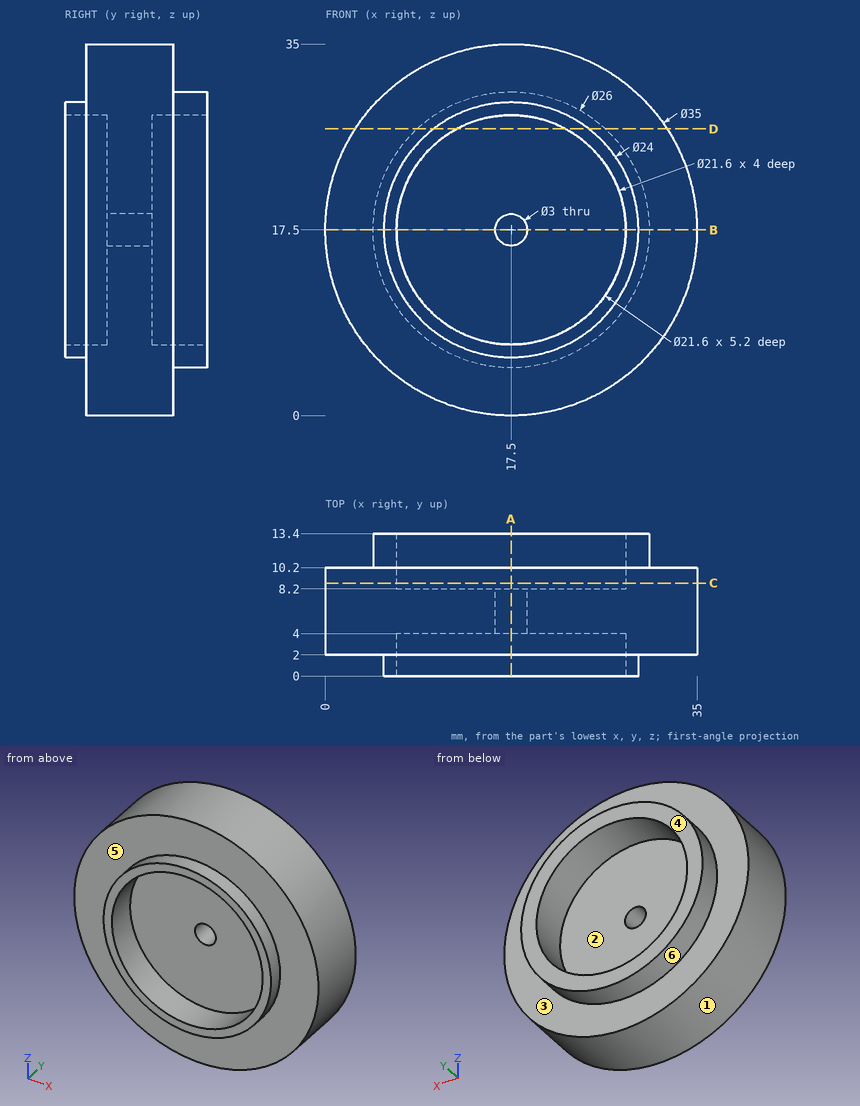
Check sheet for the drawn part. Datum: minimum x, y, z corner. Units: mm. A direction names the side the tool comes from. Round coordinates to 2 decimals unless told otherwise and drop trailing zeros. Loops run counter-clockwise (first coordinate to the right, second up) from the corner with the lowest first, then second, coordinate; pieces in that order, holes last. Notation, with made-up numbers: (54.5, 16) -> (61.5, 16) arc R21 cw to (61.5, 53) -> close; hole circle Ø2 at (60.5, 27). An arc over 180 degrees is marked (long way). Put each result on its own line as item: value. Start each with the question number.
1. Section check C-C (y = 8.75). Enter the section's corners in (x, z), plus the area to 3 significant figures.
2. Draft check along Z on the marked faces 1, 2 and 3. Enter one of: +Z half, -Z half, draft (parallel to the pull), parting line (faces both ways), or undercut.
3. Section check B-B (z = 17.5). Enter the section's corners in (x, y).
4. Section check A-A (x = 17.5). Enter the section's corners in (y, z), plus the area to 3 significant figures.
5. Access from +Z, -Z, +X, -X, +Y, -Y to the whole of each face (thin tool, end or side, straight path). Record for the marked faces 4, 5 and 6.
6. Gauge pin test, flat ends, axial feed: pin 1 (6 mm diameter, centred on y = 3.5, z = 26, fed in from +X); pin 2 (8 mm diameter, centred on x = 4.5, y = 12, fed in from -Z); pin 3 (10.5 mm diameter, centred on x = 18, z = 13.5, fed in from -Y). Record the tip position at first contact, or that the pin passes through.
7. Section check D-D (z = 27). Enter the section's corners in (x, y).
8. Scan lines: probe 1 along X at (y, z) = (7.05, 17.5); probe 2 along X at (y, z) = (1.1, 17.5); probe 3 along Y at (x, z) = (2, 12.5). Record each from-to range of solid material in increasing order.
Findings:
1. outline: circle Ø35 at (17.5, 17.5); hole circle Ø21.6 at (17.5, 17.5)
1. area: 596 mm^2
2. face 1: parting line
2. face 2: undercut
2. face 3: draft
3. outline: (0, 2) -> (5.5, 2) -> (5.5, 0) -> (6.7, 0) -> (6.7, 4) -> (16, 4) -> (16, 8.2) -> (6.7, 8.2) -> (6.7, 13.4) -> (4.5, 13.4) -> (4.5, 10.2) -> (0, 10.2) -> close; (19, 4) -> (28.3, 4) -> (28.3, 0) -> (29.5, 0) -> (29.5, 2) -> (35, 2) -> (35, 10.2) -> (30.5, 10.2) -> (30.5, 13.4) -> (28.3, 13.4) -> (28.3, 8.2) -> (19, 8.2) -> close
4. outline: (0, 5.5) -> (2, 5.5) -> (2, 0) -> (10.2, 0) -> (10.2, 4.5) -> (13.4, 4.5) -> (13.4, 6.7) -> (8.2, 6.7) -> (8.2, 16) -> (4, 16) -> (4, 6.7) -> (0, 6.7) -> close; (0, 28.3) -> (4, 28.3) -> (4, 19) -> (8.2, 19) -> (8.2, 28.3) -> (13.4, 28.3) -> (13.4, 30.5) -> (10.2, 30.5) -> (10.2, 35) -> (2, 35) -> (2, 29.5) -> (0, 29.5) -> close
4. area: 207 mm^2
5. face 4: +Z, -Z, +X, -X, +Y
5. face 5: -Y
5. face 6: +Y
6. pin 1: stops at x = 34.11
6. pin 2: stops at z = 2.76
6. pin 3: stops at y = 4
7. outline: (2.8, 2) -> (10.17, 2) -> (10.17, 0) -> (12.36, 0) -> (12.36, 4) -> (22.64, 4) -> (22.64, 0) -> (24.83, 0) -> (24.83, 2) -> (32.2, 2) -> (32.2, 10.2) -> (26.37, 10.2) -> (26.37, 13.4) -> (22.64, 13.4) -> (22.64, 8.2) -> (12.36, 8.2) -> (12.36, 13.4) -> (8.63, 13.4) -> (8.63, 10.2) -> (2.8, 10.2) -> close
8. probe 1: x = 0 to 16, 19 to 35
8. probe 2: x = 5.5 to 6.7, 28.3 to 29.5
8. probe 3: y = 2 to 10.2
